Job drawing, mm, ordinate dimensions from the low corner. One solid piece. A direction names the side the tool comes from. Give positions to 0.01 mm unless a question says otherwise; leave off trailing zeros. Write each loop counter-clockwise with the first axis right and the second up, starting at its lowest first coordinate (ties: lowest second). Pieces come first, ordered by that corner, then holes. Notation, with made-up numbers: M -4.75,76.5 L 22.25,76.5 A18 ccw 22.25,93.5 Z; hole C -10,-15.75 d10. An arc over 180 degrees is marked long. Use a Markdown table: item, result.
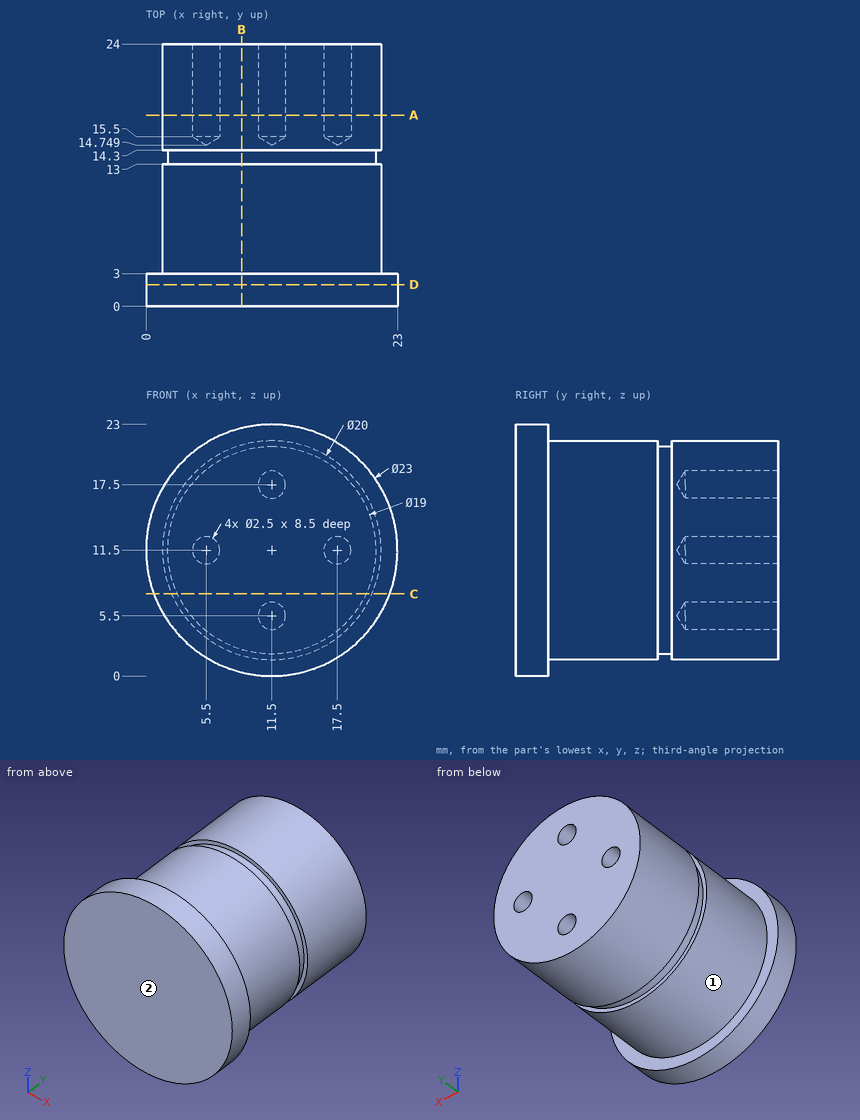
1. Cut at D-D, the plane y = 2. Give the cut face in (x, z), then the cut area to 3 significant figures.
Findings below:
| item | result |
|---|---|
| outline | C 11.5,11.5 d23 |
| area | 415 mm2 |
2. Drop flat-ended pins along their axis: P1, Ø10, axis at y = 18, z = 11, coming from the +X side; P2, Ø1.5, axis at x = 11.5, z = 17.5, coming from the +Y side; P3, Ø8, axis at y = 8, z = 18.5, coming from the +X side. Give the stop position or say it passes through.
Findings below:
| item | result |
|---|---|
| P1 | x = 21.5 |
| P2 | y = 15.2 |
| P3 | x = 21.04 |
3. Tool access for the marked faces 1 and 2: list every direction of +Z, -Z, +X, -X, +Y, -Y with a clear straight run to the whole face (end or side of a thin tool).
Findings below:
| item | result |
|---|---|
| face 1 | +Y |
| face 2 | +Z, -Z, +X, -X, -Y |
4. Cut at B-B, the plane x = 8.75. Give the cut face in (y, z), then the cut area to 3 significant figures.
Findings below:
| item | result |
|---|---|
| outline | M 0,0.33 L 3,0.33 L 3,1.89 L 13,1.89 L 13,2.41 L 14.3,2.41 L 14.3,1.89 L 24,1.89 L 24,21.11 L 14.3,21.11 L 14.3,20.59 L 13,20.59 L 13,21.11 L 3,21.11 L 3,22.67 L 0,22.67 Z |
| area | 469 mm2 |
5. Drill centre lines: L1, parallel to X at y = 21.5, z = 11.5; L2, parallel to Y at x = 7.5, z = 21.75; L3, parallel to X at y = 17.5, z = 5.5. Where is each one in solid material? Low to high.
Findings below:
| item | result |
|---|---|
| L1 | 1.5 to 4.25, 6.75 to 16.25, 18.75 to 21.5 |
| L2 | 0 to 3 |
| L3 | 3.5 to 10.25, 12.75 to 19.5 |
6. Cut at C-C, the plane z = 7.5. Give the cut face in (x, y) (3 decimals), then the cut area to 3 significant figures.
Findings below:
| item | result |
|---|---|
| outline | M 0.718,0 L 22.282,0 L 22.282,3 L 20.665,3 L 20.665,13 L 20.117,13 L 20.117,14.3 L 20.665,14.3 L 20.665,24 L 2.335,24 L 2.335,14.3 L 2.883,14.3 L 2.883,13 L 2.335,13 L 2.335,3 L 0.718,3 Z |
| area | 448 mm2 |
7. Cut at A-A, the plane y = 17.5. Give the cut face in (x, z).
Findings below:
| item | result |
|---|---|
| outline | C 11.5,11.5 d20; hole C 5.5,11.5 d2.5; hole C 11.5,5.5 d2.5; hole C 11.5,17.5 d2.5; hole C 17.5,11.5 d2.5 |
